from build123d import *

# Parameters (mm, degrees)
SKETCH_1_W          = 40
SKETCH_1_H          = 20
SKETCH_1_W_2        = 38
SKETCH_1_H_2        = 18
EXTRUDE_1_DEPTH     = 550
SKETCH_4_R          = 1.75
CUT_EXTRUDE_2_DEPTH = 1.5


with BuildPart() as part:
    # 草图1 → 拉伸-薄壁1 (new body)
    with BuildSketch(Plane.XY):
        with Locations((20, -10)):
            Rectangle(SKETCH_1_W, SKETCH_1_H)
        with Locations((20, -10)):
            Rectangle(SKETCH_1_W_2, SKETCH_1_H_2, mode=Mode.SUBTRACT)
    extrude(amount=EXTRUDE_1_DEPTH)

    # 草图4 → 切除-拉伸2 (cut)
    with BuildSketch(Plane.ZY):
        with Locations((539.996387591, -10)):
            Circle(SKETCH_4_R)
        with Locations((10, -10.000000002)):
            Circle(SKETCH_4_R)
    extrude(amount=-CUT_EXTRUDE_2_DEPTH, mode=Mode.SUBTRACT)


solid = part.part
Read the model definition and answer for the solid it produces. Units are mm, in the model's axes. A direction names the side the tool comes from. Coordinates: 2 decimals unless noted, no trailing zeros. Loops run counter-clockwise (first coordinate to the right, second up) from the corner with the lowest first, then second, coordinate; pieces in that order, holes last. Notation, with made-up numbers: (79, 69) -> (87, 69) arc R30 ccw to (87, 105) -> close; hole circle Ø6 at (33, 73). An arc over 180 degrees is marked (long way). Answer in a Markdown table with one row per item.
Item 1: Straight lines are drawn through the part: line 1 along Y through (x, z) = (37.5, 316.5); line 2 along X through (y, z) = (-13.75, 186); line 3 along Y through (x, z) = (0.75, 10). For each, find the intervals that lie inside material, in ascending order. Write a range as [from, to].
Returned:
| item | result |
|---|---|
| line 1 | y = [-20, -19], [-1, 0] |
| line 2 | x = [0, 1], [39, 40] |
| line 3 | y = [-20, -11.75], [-8.25, 0] |
Item 2: A cutting plane is placed at A-A on y = -5. Determine the outline of the cut face in (x, z), plus the area to 3 significant figures.
Returned:
| item | result |
|---|---|
| outline | (0, 0) -> (1, 0) -> (1, 550) -> (0, 550) -> close; (39, 0) -> (40, 0) -> (40, 550) -> (39, 550) -> close |
| area | 1,100 mm^2 |
Item 3: A cutting plane is placed at B-B on z = 506. Determine the outline of the cut face in (x, y), plus the area to 3 significant figures.
Returned:
| item | result |
|---|---|
| outline | (0, -20) -> (40, -20) -> (40, 0) -> (0, 0) -> close; hole (1, -19) -> (39, -19) -> (39, -1) -> (1, -1) -> close |
| area | 116 mm^2 |
Item 4: For faces 4 (the flat face through (18.4, -19.6, 0)), 5 (the flat face through (20, -19, 271)), determine the directions among +Z, -Z, +X, -X, +Y, -Y from which every point of the face is accessible in a straight line to the end or side of a thin tool.
Returned:
| item | result |
|---|---|
| face 4 | -Z, +X, -X, +Y, -Y |
| face 5 | +Z, -Z |
Item 5: For a pull along X with two mould halves and no side action, classify faces 1 (the flat face through (20, -20, 271)), 2 (the flat face through (39, -10, 271)), 3 (the flat face through (40, -10, 271)) as released by +X, released by -X, zero draft, split by the parting line, or undercut.
Returned:
| item | result |
|---|---|
| face 1 | zero draft |
| face 2 | undercut |
| face 3 | released by +X |
Item 6: A cutting plane is placed at C-C on x = 22. Determine the outline of the cut face in (y, z).
Returned:
| item | result |
|---|---|
| outline | (-20, 0) -> (-19, 0) -> (-19, 550) -> (-20, 550) -> close; (-1, 0) -> (0, 0) -> (0, 550) -> (-1, 550) -> close |
